```python
from build123d import *

# Parameters (mm, degrees)
SKETCH1_R           = 3
BOSS_EXTRUDE1_DEPTH = 30
FILLET1_R           = 2


with BuildPart() as part:
    # Sketch1 → Boss-Extrude1 (new body)
    with BuildSketch(Plane(origin=(0, 0, 0), x_dir=(1, 0, 0), z_dir=(0, 1, 0))):
        with BuildLine():
            Line((120, 0), (-0.016209805, 6.346913517))
            ThreePointArc((-0.016209805, 6.346913517), (-6.346913517, -0.016209805), (0.016209805, -6.346913517))
            Line((0.016209805, -6.346913517), (120, 0))
        make_face()
        with Locations(Location((0, 0, 0), (0, 0, 270))):
            Circle(SKETCH1_R, mode=Mode.SUBTRACT)
    extrude(amount=BOSS_EXTRUDE1_DEPTH)

    # Fillet1
    fillet1_edges = [part.edges().sort_by_distance(p)[0] for p in [
        (120, 15, 0),
    ]]
    fillet(fillet1_edges, radius=FILLET1_R)


solid = part.part
```
For this review, take the finished solid that the model builds, in its own axes (mm). Round coordinates to 2 decimals unless told otherwise and drop trailing zeros. Write each loop counter-clockwise with the first axis right and the second up, starting at its lowest first coordinate (ties: lowest second). Pieces come first, ordered by that corner, then holes. Notation, with made-up numbers: M 84.25,-34.75 L 131.25,-34.75 A21 cw 131.25,-19.75 Z; hole C -13,22.25 d7. An arc over 180 degrees is marked long. One line per item, written item: value. Start each with the question number.
(1) We need section D-D (x = 67). Give the boundary of the cut face in (y, z), and give its area (3 significant figures).
(2) Wall thickness on line 1 (X direction, y = 11, z = -1.5); line 2 (X direction, y = 9, z = 0); line 3 (Z direction, x = -1, y = 3.25): over which ranges is each line inside the solid? List them lowest first.
(3) The part is to be moulded in two halves that separate along Z. For faces 1 (the flat face through (40.6, 14.8, 4.2)), 2 (the flat face through (28, 0, 0)), 3 (the cylindrical face through (84.133, 15.21, -0.042)), 4 (the cylindrical face through (0.9, 14.79, 2.86)), say which applies: released by +Z, released by -Z, zero draft, split by the parting line, or undercut.
(4) We need section A-A (z = 0). Give the boundary of the cut face in (x, y).
(5) We need section C-C (y = 20.25). Give the boundary of the cut face in (x, z).
(6) Insertion check: pin 1 (6 mm diameter, centred on x = 59.5, y = 20, fed in from -Z); pin 2 (5 mm diameter, centred on x = 26.5, y = 16, fed in from +Z); pin 3 (2 mm diameter, centred on x = 67, y = 21.5, fed in from -Z). Each pin has a flat end and moves straight along its axis. Give the tip position at first contact, or say it passes through.
(7) We need section B-B (x = 2). Give the boundary of the cut face in (y, z).
Result:
1. outline: M 0,-2.8 L 30,-2.8 L 30,2.8 L 0,2.8 Z
1. area: 168 mm²
2. line 1: -6.17 to -2.6, 2.6 to 83.46
2. line 2: -6.35 to -3, 3 to 84.13
2. line 3: -6.27 to -2.83, 2.83 to 6.27
3. face 1: released by +Z
3. face 2: zero draft
3. face 3: split by the parting line
3. face 4: undercut
4. outline: M -6.35,0 L -3,0 L -3,30 L -6.35,30 Z; M 3,0 L 84.13,0 L 84.13,30 L 3,30 Z
5. outline: M -0.02,-6.35 L 82.24,-2 A2 ccw 82.24,2 L 0.02,6.35 A6.35 ccw Z; hole C 0,0 d6
6. pin 1: z = -3.36
6. pin 2: z = 5.08
6. pin 3: z = -2.86
7. outline: M 0,-6.24 L 30,-6.24 L 30,-2.24 L 0,-2.24 Z; M 0,2.24 L 30,2.24 L 30,6.24 L 0,6.24 Z
